from build123d import *

# Parameters (mm, degrees)
SKETCH006_W     = 5
SKETCH006_H     = 6
SKETCH006_W_2   = 10
SKETCH006_H_2   = 7
SKETCH006_W_3   = 2.5
SKETCH006_H_3   = 1.5
PAD002_DEPTH    = 8
SKETCH007_R     = 15
POCKET004_DEPTH = 8.001
SKETCH008_W     = 2.5
SKETCH008_H     = 4.49
POCKET005_DEPTH = 4.251
SKETCH009_W     = 3.873062
SKETCH009_H     = 0.5
POCKET006_DEPTH = 6.501


with BuildPart() as part:
    # Sketch006 → Pad002 (new body)
    with BuildSketch(Plane.XZ):
        with Locations((-16.07, 0)):
            Rectangle(SKETCH006_W, SKETCH006_H)
        with Locations((-23.57, 0)):
            Rectangle(SKETCH006_W_2, SKETCH006_H_2)
        with Locations((-29.82, 0)):
            Rectangle(SKETCH006_W_3, SKETCH006_H_3)
    extrude(amount=PAD002_DEPTH)

    # Sketch007 (on Face14 of Pad002) → Pocket004 (cut, through all)
    with BuildSketch(Plane.XZ.offset(8)):
        Circle(SKETCH007_R)
    extrude(amount=-POCKET004_DEPTH, mode=Mode.SUBTRACT)

    # Sketch008 (on Face8 of Pocket004) → Pocket005 (cut, through all)
    with BuildSketch(Plane(origin=(0, 0, 0.75), x_dir=(-1, 0, 0), z_dir=(0, 0, 1))):
        with Locations((29.82, 5.755)):
            Rectangle(SKETCH008_W, SKETCH008_H)
        with Locations((29.82, 2.245)):
            Rectangle(SKETCH008_W, SKETCH008_H)
    extrude(amount=-POCKET005_DEPTH, mode=Mode.SUBTRACT)

    # Sketch009 (on Face8 of Pocket005) → Pocket006 (cut, through all)
    with BuildSketch(Plane(origin=(0, 0, 3), x_dir=(-1, 0, 0), z_dir=(0, 0, 1))):
        with Locations((16.633469, 7.75)):
            Rectangle(SKETCH009_W, SKETCH009_H)
        with Locations((16.633469, 0.25)):
            Rectangle(SKETCH009_W, SKETCH009_H)
    extrude(amount=-POCKET006_DEPTH, mode=Mode.SUBTRACT)


with BuildPart() as part_1:
    # Body002 placement: moved
    add(part.part.moved(Location((0, 15, 0))))


solid = part_1.part
CAD build for the part. Positions are in the model's coordinates, mm. A direction names the side the tool comes from. Coordinates: 2 decimals unless noted, no trailing zeros. Order: outer loops, then holes, each group sorted by start corner. A loop starts at its lowest first (then second) coordinate and runs counter-clockwise, first axis right, second up.
Item 1: 3-axis set-ups, long thin cutter, end or side, ignore diameter. For faces 1 (the face through (-17, 7.5, 0)), 2 (the face through (-24, 11, 3.5)), 3 (the face through (-24, 15, 0)), 4 (the face through (-17, 14.5, 0)), 5 (the face through (-17, 11, -3)): which of +Z, -Z, +X, -X, +Y, -Y reach the whole face in a straight line?
Check sheet entries:
face 1: +Z, -Z, +X, -Y
face 2: +Z, +X, -X, +Y, -Y
face 3: +Z, -Z, +X, -X, +Y
face 4: +Z, -Z, +X, +Y
face 5: -Z, +X, +Y, -Y
Item 2: Band-saw the part on B-B on z = 0. List the corners of the cut face in (x, y), plus the area to 3 significant figures.
Check sheet entries:
outline: (-28.57, 7) - (-18.57, 7) - (-18.57, 7.5) - (-15, 7.5) - (-15, 14.5) - (-18.57, 14.5) - (-18.57, 15) - (-28.57, 15) - close
area: 105 mm2
Item 3: Drill centre lines: L1, parallel to Z at x = -18.25, y = 12; L2, parallel to Y at x = -17, z = 0; L3, parallel to X at y = 12.5, z = 3.25. Where is each one in solid material? Low to high.
Check sheet entries:
L1: z = -3 to 3
L2: y = 7.5 to 14.5
L3: x = -28.57 to -18.57
Item 4: Pin check, flat tips, straight feed: pin 1 Ø3 at (x, y) = (-17, 12.5) entering from +Z; pin 2 Ø1 at (x, y) = (-17.5, 10) entering from -Z; pin 3 Ø1 at (y, z) = (8.5, 1.5) entering from +X. Stop position of each tip, or through.
Check sheet entries:
pin 1: stops at z = 3
pin 2: stops at z = -3
pin 3: stops at x = -14.87
Item 5: Band-saw the part on C-C on x = -16.75. List the corners of the cut face in (y, z), plus the area to 3 significant figures.
Check sheet entries:
outline: (7.5, -3) - (14.5, -3) - (14.5, 3) - (7.5, 3) - close
area: 42.0 mm2
Item 6: Band-saw the part on A-A on y = 13.5. List the corners of the cut face in (x, z), plus the area to 3 significant figures.
Check sheet entries:
outline: (-28.57, -3.5) - (-18.57, -3.5) - (-18.57, -3) - (-14.7, -3) arc R15 cw to (-14.7, 3) - (-18.57, 3) - (-18.57, 3.5) - (-28.57, 3.5) - close
area: 92.0 mm2
Item 7: Two-plate mould, pull along Z, no slides. Class faces 6 (the face through (-15, 11, 0)), 7 (the face through (-17, 11, 3)), 8 (the face through (-28.57, 11, 0)), 9 (the face through (-24, 11, -3.5)): +Z half, -Z half, draft (parallel to the pull), parting line (faces both ways), or undercut.
Check sheet entries:
face 6: undercut
face 7: +Z half
face 8: draft
face 9: -Z half
Item 8: Band-saw the part on D-D on y = 14.75. List the corners of the cut face in (x, z), plus the area to 3 significant figures.
Check sheet entries:
outline: (-28.57, -3.5) - (-18.57, -3.5) - (-18.57, 3.5) - (-28.57, 3.5) - close
area: 70.0 mm2
